```python
from build123d import *

# Parameters (mm, degrees)
SKETCH1_R           = 2.1082
SKETCH1_R_2         = 2.2
BOSS_EXTRUDE1_DEPTH = 4.5


with BuildPart() as part:
    # Sketch1 → Boss-Extrude1 (new body)
    with BuildSketch(Plane(origin=(0, 0, 0), x_dir=(1, 0, 0), z_dir=(0, 1, 0))):
        with BuildLine():
            Line((55.75, 16.51), (22.65807516, 16.51))
            ThreePointArc((22.65807516, 16.51), (21.243861598, 15.924213562), (20.65807516, 14.51))
            Line((20.65807516, 14.51), (20.65807516, -8.345000078))
            Line((20.65807516, -8.345000078), (-20.38832484, -8.345000078))
            Line((-20.38832484, -8.345000078), (-20.38832484, 14.51))
            ThreePointArc((-20.38832484, 14.51), (-20.974111278, 15.924213562), (-22.38832484, 16.51))
            Line((-22.38832484, 16.51), (-55.75, 16.51))
            ThreePointArc((-55.75, 16.51), (-57.164213562, 15.924213562), (-57.75, 14.51))
            Line((-57.75, 14.51), (-57.75, -14.51))
            ThreePointArc((-57.75, -14.51), (-57.164213562, -15.924213562), (-55.75, -16.51))
            Line((-55.75, -16.51), (55.75, -16.51))
            ThreePointArc((55.75, -16.51), (57.164213562, -15.924213562), (57.75, -14.51))
            Line((57.75, -14.51), (57.75, 14.51))
            ThreePointArc((57.75, 14.51), (57.164213562, 15.924213562), (55.75, 16.51))
        make_face()
        with Locations(Location((-37.20312484, 1.689999922, 0), (0, 0, 270))):
            Circle(SKETCH1_R, mode=Mode.SUBTRACT)
        with Locations(Location((50.40147516, 1.689999922, 0), (0, 0, 90))):
            Circle(SKETCH1_R, mode=Mode.SUBTRACT)
        with Locations(Location((-23.988324752, 6.404999922, 0), (0, 0, 270))):
            Circle(SKETCH1_R_2, mode=Mode.SUBTRACT)
        with Locations(Location((24.258075072, 6.404999922, 0), (0, 0, 90))):
            Circle(SKETCH1_R_2, mode=Mode.SUBTRACT)
        with Locations(Location((24.258075072, -3.025000078, 0), (0, 0, 270))):
            Circle(SKETCH1_R_2, mode=Mode.SUBTRACT)
        with Locations(Location((-23.988324752, -3.025000078, 0), (0, 0, 90))):
            Circle(SKETCH1_R_2, mode=Mode.SUBTRACT)
    extrude(amount=BOSS_EXTRUDE1_DEPTH)


solid = part.part
```
Check sheet for the modelled part. Datum: model origin and axes. Units: mm. A direction names the side the tool comes from. Give positions to 0.01 mm unless a question says otherwise; leave off trailing zeros. Order: outer loops, then holes, each group sorted by start corner. A loop starts at its lowest first (then second) coordinate and runs counter-clockwise, first axis right, second up. Notation, with made-up numbers: (-1.75, 0.25) -> (40.25, 0.25) arc R16 ccw to (40.25, 17.25) -> close; hole circle Ø10 at (29, -17). An arc over 180 degrees is marked (long way). Use CSV: the item, a comma, the result in double quotes. Start each with the question number.
1) Sectioned sample at A-A, the plane z = -11. Record the boundary of the cut face in (x, y), plus the area to 3 significant figures.
2) Go/stop test with a flat-tipped pin: P1, Ø2.5, axis at x = 24.26, z = -6.4, coming from the +Y side. Record where the tip stops, or that it passes through.
3) Sectioned sample at C-C, the plane y = 1.3. Record the boundary of the cut face in (x, z) (3 decimals).
4) Sectioned sample at B-B, the plane z = -1.69. Record the boundary of the cut face in (x, y), plus the area to 3 significant figures.
5) Material ranges on line 1 (X direction, y = 2.05, z = -1.69); line 2 (X direction, y = 3.4, z = 1); line 3 (Z direction, x = -24, y = 3.4), recorded low to high. Write a range as from..to.
6) Set-up check for faces 1 (the face through (-20.96, 2.22, -15.91)), 2 (the face through (22.771, 2.218, -4.784)): record each of +Z, -Z, +X, -X, +Y, -Y from which the full face is reachable in a straight line by a thin tool's end or side.
7) Sectioned sample at D-D, the plane z = 4. Record the boundary of the cut face in (x, y), plus the area to 3 significant figures.
8) Mould release check, pull along X, two halves, no side actions. Record for faces 3 (the face through (-1, 0, 11)), 4 (the face through (21.26, 2.22, -15.94)), 5 (the face through (57.15, 2.22, 15.94)): released by +X, released by -X, zero draft, split by the parting line, or undercut.
Recorded:
1,outline,"(-57.75, 0) -> (-20.39, 0) -> (-20.39, 4.5) -> (-57.75, 4.5) -> close; (20.66, 0) -> (57.75, 0) -> (57.75, 4.5) -> (20.66, 4.5) -> close"
1,area,"335 mm2"
2,P1,"through"
3,outline,"(-57.75, -14.51) arc R2 ccw to (-55.75, -16.51) -> (-22.388, -16.51) arc R2 ccw to (-20.388, -14.51) -> (-20.388, 8.345) -> (20.658, 8.345) -> (20.658, -14.51) arc R2 ccw to (22.658, -16.51) -> (55.75, -16.51) arc R2 ccw to (57.75, -14.51) -> (57.75, 14.51) arc R2 ccw to (55.75, 16.51) -> (-55.75, 16.51) arc R2 ccw to (-57.75, 14.51) -> close; hole circle Ø4.216 at (-37.203, -1.69); hole circle Ø4.4 at (-23.988, -6.405); hole circle Ø4.4 at (-23.988, 3.025); hole circle Ø4.4 at (24.258, -6.405); hole circle Ø4.4 at (24.258, 3.025); hole circle Ø4.216 at (50.401, -1.69)"
4,outline,"(-57.75, 0) -> (-39.31, 0) -> (-39.31, 4.5) -> (-57.75, 4.5) -> close; (-35.09, 0) -> (-20.39, 0) -> (-20.39, 4.5) -> (-35.09, 4.5) -> close; (20.66, 0) -> (48.29, 0) -> (48.29, 4.5) -> (20.66, 4.5) -> close; (52.51, 0) -> (57.75, 0) -> (57.75, 4.5) -> (52.51, 4.5) -> close"
4,area,"297 mm2"
5,line 1,"-57.75..-39.31, -35.09..-20.39, 20.66..48.29, 52.51..57.75"
5,line 2,"-57.75..-24.85, -23.13..-20.39, 20.66..23.4, 25.12..57.75"
5,line 3,"-16.51..-8.6, -4.21..0.83, 5.22..16.51"
6,face 1,"-Z, +Y, -Y"
6,face 2,"+Y, -Y"
7,outline,"(-57.75, 0) -> (-25.96, 0) -> (-25.96, 4.5) -> (-57.75, 4.5) -> close; (-22.02, 0) -> (-20.39, 0) -> (-20.39, 4.5) -> (-22.02, 4.5) -> close; (20.66, 0) -> (22.29, 0) -> (22.29, 4.5) -> (20.66, 4.5) -> close; (26.23, 0) -> (57.75, 0) -> (57.75, 4.5) -> (26.23, 4.5) -> close"
7,area,"300 mm2"
8,face 3,"zero draft"
8,face 4,"undercut"
8,face 5,"released by +X"
